Check sheet for the drawn part. Datum: minimum x, y, z corner. Units: mm. A direction names the side the tool comes from. Coordinates: 2 decimals unless noted, no trailing zeros. Order: outer loops, then holes, each group sorted by start corner. A loop starts at its lowest first (then second) coordinate and runs counter-clockwise, first axis right, second up.
Q1. Cross-section at B-B, the plane z = 54.8. Record the boundary of the cut face in (x, y).
Q2. Cross-section at D-D, the plane y = 23.75. Record the boundary of the cut face in (x, z), and give its area (3 significant figures).
Q3. Cross-section at A-A, the plane y = 17. Record the boundary of the cut face in (x, z).
Q4. Depth check by flat-ended pin: P1, Ø1.6, axis at y = 13.875, z = 36.3, coming from the +X side; P2, Ø2.5, axis at x = 20, y = 17, coming from the -Z side; P3, Ø5.5, axis at x = 12.5, y = 19, coming from the +Z side; P4, Ø9.5, axis at y = 15, z = 66, coming from the +X side. Enter the tip coordinate at first touch or a pass-through.
Q5. Set-up check for the marked faces 1 and 2: record each of +Z, -Z, +X, -X, +Y, -Y from which the full face is reachable in a straight line by a thin tool's end or side.
Q6. Cross-section at C-C, the plane x = 22. Record the boundary of the cut face in (y, z) (3 decimals), and give its area (3 significant figures).
Q7. Thickness scan on line 1 (Y direction, x = 20, z = 55.95); line 2 (Z direction, x = 21.1, y = 17); line 3 (Z direction, x = 19.25, y = 23). Record the ranges inside material, lowest first.
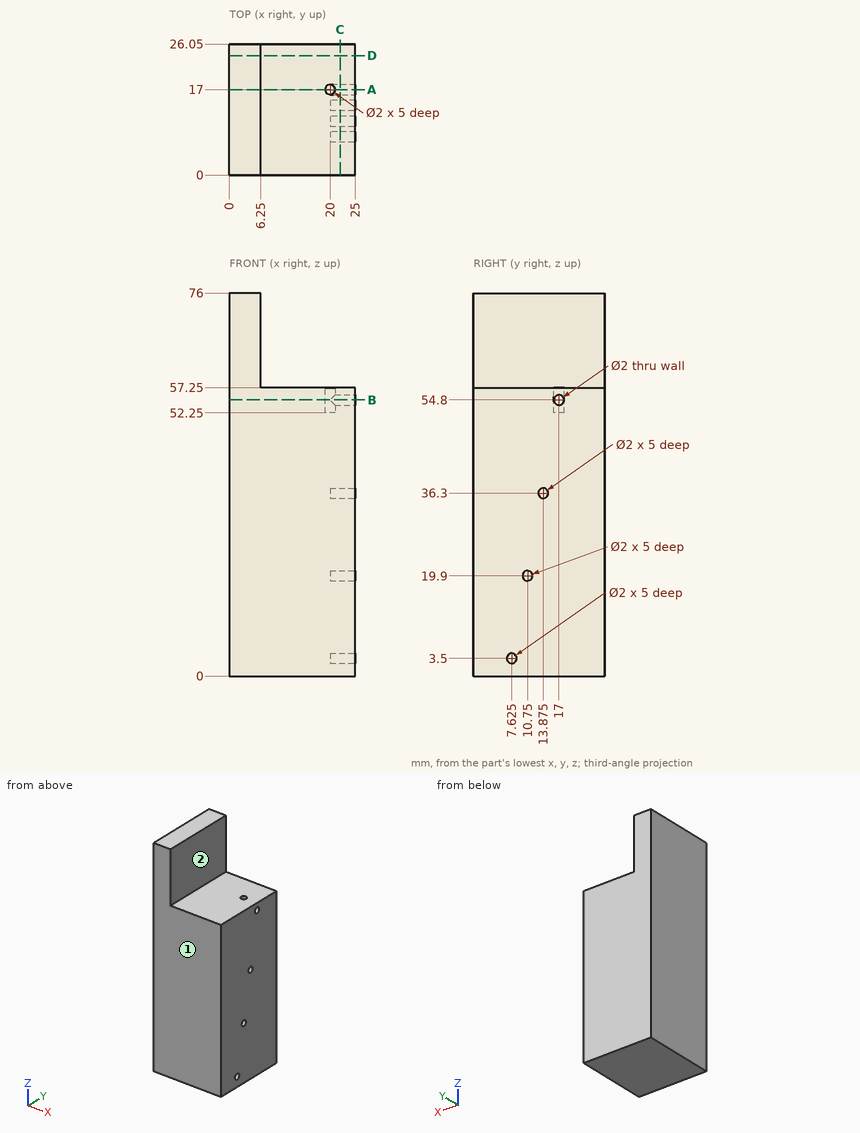
Check values:
1. outline: (0, 0) - (25, 0) - (25, 16) - (20, 16) arc R1 cw to (20, 18) - (25, 18) - (25, 26.05) - (0, 26.05) - close
2. outline: (0, 0) - (25, 0) - (25, 57.25) - (6.25, 57.25) - (6.25, 76) - (0, 76) - close
2. area: 1,550 mm2
3. outline: (0, 0) - (25, 0) - (25, 53.8) - (21, 53.8) - (21, 52.25) - (19, 52.25) - (19, 57.25) - (6.25, 57.25) - (6.25, 76) - (0, 76) - close; (21, 55.8) - (25, 55.8) - (25, 57.25) - (21, 57.25) - close
4. P1: stops at x = 20
4. P2: stops at z = 0
4. P3: stops at z = 57.25
4. P4: stops at x = 6.25
5. face 1: +Z, -Z, +X, -X, -Y
5. face 2: +Z, +X, +Y, -Y
6. outline: (0, 0) - (26.05, 0) - (26.05, 57.25) - (0, 57.25) - close; hole circle Ø2 at (7.625, 3.5); hole circle Ø2 at (10.75, 19.9); hole circle Ø2 at (13.875, 36.3); hole circle Ø2 at (17, 54.8)
6. area: 1,480 mm2
7. line 1: y = 0 to 16, 18 to 26.05
7. line 2: z = 0 to 53.8, 55.8 to 57.25
7. line 3: z = 0 to 57.25
